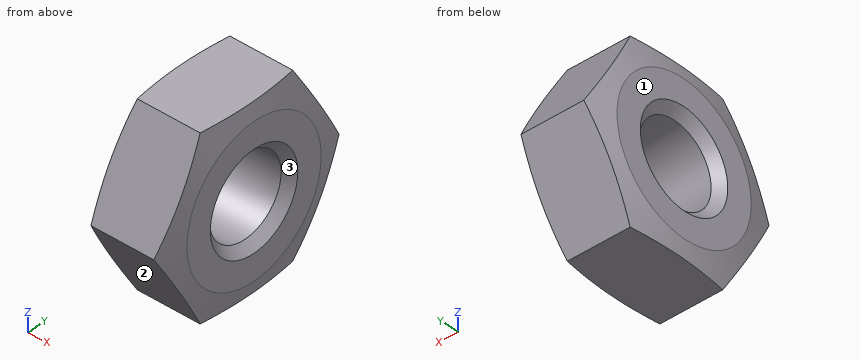
Solid Edge part; units mm, degrees
sketch "Sketch1" plane through (0, 0, 0) normal (0, -1, 0) x (1, 0, 0)
  line L0 (0, 0) -> (0, -2.3)
  line L1 (0, -2.3) -> (0.2679, -3.3)
  line L2 (0.2679, -3.3) -> (2.1321, -3.3)
  line L3 (2.1321, -3.3) -> (2.4, -2.3)
  line L4 (2.4, -2.3) -> (2.4, 0)
  line L5 (2.4, 0) -> (0, 0)
revolve "RevolvedProtrusion1" add sketch "Sketch1" angle 360 about axis through (2.4, 0, 0) along (-1, 0, 0)
sketch "Sketch2" plane through (0, 0, 0) normal (1, 0, 0) x (0, 1, 0)
  line L0 (11, 11) -> (-11, 11)
  line L1 (-11, 11) -> (-11, -11)
  line L2 (-11, -11) -> (11, -11)
  line L3 (11, -11) -> (11, 11)
  line L4 (1.5877, 2.75) -> (-1.5877, 2.75)
  line L5 (-1.5877, 2.75) -> (-3.1754, 0)
  line L6 (-3.1754, 0) -> (-1.5877, -2.75)
  line L7 (-1.5877, -2.75) -> (1.5877, -2.75)
  line L8 (1.5877, -2.75) -> (3.1754, 0)
  line L9 (3.1754, 0) -> (1.5877, 2.75)
extrude "ExtrudedCutout_1" cut sketch "Sketch2" against normal blind 3.4 and the other way blind 3.4
sketch "Sketch3" plane through (0, 0, 0) normal (0, 0, 1) x (1, 0, 0)
  line L0 (0, 0) -> (0, 1.5)
  line L1 (0, 1.5) -> (0.2705, 1.2295)
  line L2 (0.2705, 1.2295) -> (2.1295, 1.2295)
  line L3 (2.1295, 1.2295) -> (2.4, 1.5)
  line L4 (2.4, 1.5) -> (2.4, 0)
  line L5 (2.4, 0) -> (0, 0)
revolve "RevolvedCutout1" cut sketch "Sketch3" angle 360 about axis through (2.4, 0, 0) along (-1, 0, 0)
cosmetic_thread "Thread1"
properties part number "Hexagon nut - style 1 JIS B 1181 M3"
Design review of the part built by this model. Coordinates are the model's own, in mm. Face numbers are marked on the shaded views. Give positions to 0.01 mm unless a question says otherwise; leave off trailing zeros. Order: outer loops, then holes, each group sorted by start corner. A loop starts at its lowest first (then second) coordinate and runs counter-clockwise, first axis right, second up. Notation, with made-up numbers: (-21.75, 49.25) -> (-4.75, 49.25) arc R23 cw to (-4.75, 87.25) -> close; hole circle Ø10 at (33, 8.5). An arc over 180 degrees is marked (long way). Write item = value, one per line. Start each with the question number.
(1) We need section A-A on y = 0. Write out the cut boundary in (x, z), plus the area to 3 significant figures.
(2) Mouldability with a two-part tool opening along Z and no side actions: class the marked faces 1, 2 and 3 as +Z half, -Z half, draft (parallel to the pull), parting line (faces both ways), or undercut.
(3) We need section B-B on x = 0.75. Write out the cut boundary in (y, z), plus the area to 3 significant figures.
(4) To check wall thickness, follow line 1 along Z through (x, y) = (1.1, 0); line 2 along Z through (x, y) = (1.2, 0.5); line 3 along Y through (x, z) = (0.4, 0.9). State the ranges of each line that lie inside material, in increasing order.
Numbers:
q1.outline = (0, -2.3) -> (0.12, -2.75) -> (2.28, -2.75) -> (2.4, -2.3) -> (2.4, -1.5) -> (2.13, -1.23) -> (0.27, -1.23) -> (0, -1.5) -> close; (0, 1.5) -> (0.27, 1.23) -> (2.13, 1.23) -> (2.4, 1.5) -> (2.4, 2.3) -> (2.28, 2.75) -> (0.12, 2.75) -> (0, 2.3) -> close
q1.area = 7.04 mm^2
q2.face_1 = draft
q2.face_2 = -Z half
q2.face_3 = undercut
q3.outline = (-3.18, 0) -> (-1.59, -2.75) -> (1.59, -2.75) -> (3.18, 0) -> (1.59, 2.75) -> (-1.59, 2.75) -> close; hole circle Ø2.46 at (0, 0)
q3.area = 21.4 mm^2
q4.line_1 = -2.75 to -1.23, 1.23 to 2.75
q4.line_2 = -2.75 to -1.12, 1.12 to 2.75
q4.line_3 = -2.66 to -0.84, 0.84 to 2.66
